The drawing under review shows one solid part. Ordinate dimensions are in mm from its lowest x, y, z. Coordinates: 2 decimals unless noted, no trailing zeros. Write each loop counter-clockwise with the first axis right and the second up, starting at its lowest first coordinate (ties: lowest second). Pieces come first, ordered by that corner, then holes. Notation, with made-up numbers: (61, 72.25) -> (79, 72.25) arc R21 cw to (79, 110.25) -> close; hole circle Ø1 at (-3, 30.5). An arc over 180 degrees is marked (long way). One line per item, written item: value. Start each with the question number.
1) Add section A-A (x = 10). State the section outline as (y, z) points.
2) Add section C-C (z = 33). State the section outline as (x, y) points.
3) For probe 1 along Z at (x, y) = (27, 0.2); probe 2 along Z at (x, y) = (37, 0.15); probe 3 along X at (y, z) = (1.9, 15.5), list the stretches that pass through material, from the lowest coordinate up. Write a range as from..to.
4) Add section B-B (y = 0.55). State the section outline as (x, z) points.
5) For pin 1 Ø0.6 at (x, y) = (12, 1) entering from -Z, flat-tipped, find the tip position at first contact; note if it passes through.
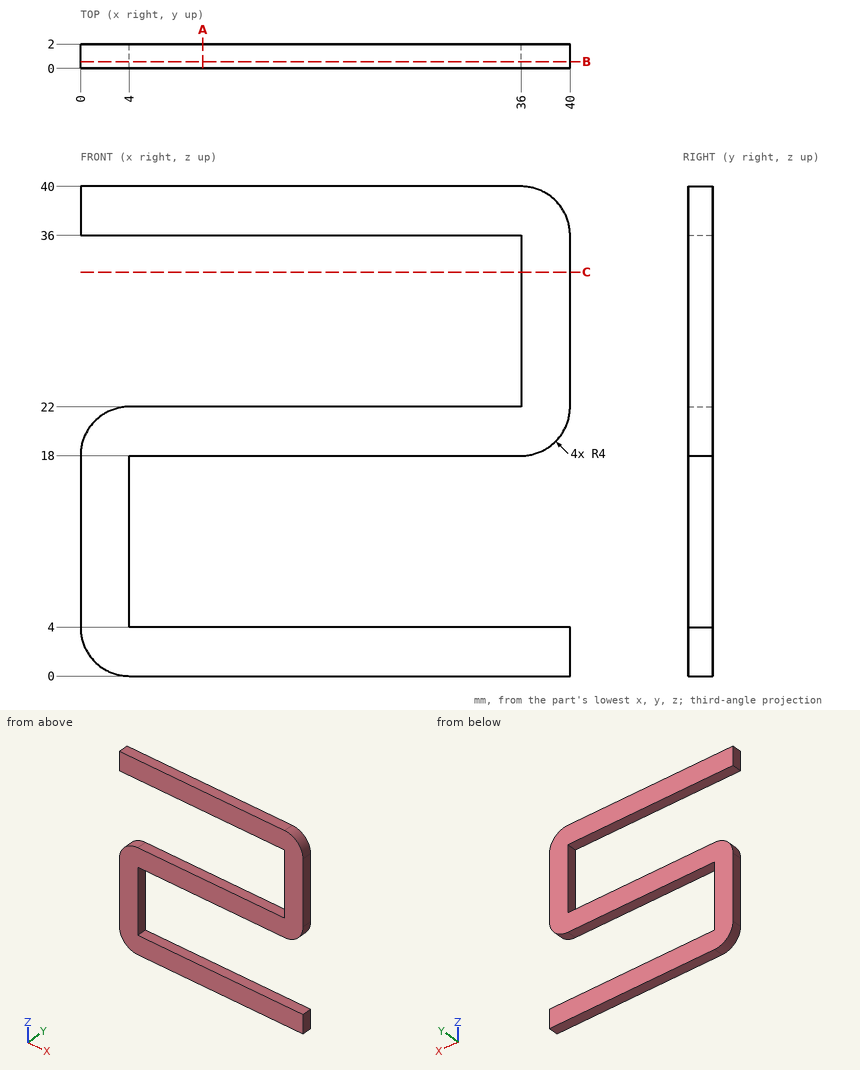
Numbers:
1. outline: (0, 0) -> (2, 0) -> (2, 4) -> (0, 4) -> close; (0, 18) -> (2, 18) -> (2, 22) -> (0, 22) -> close; (0, 36) -> (2, 36) -> (2, 40) -> (0, 40) -> close
2. outline: (36, 0) -> (40, 0) -> (40, 2) -> (36, 2) -> close
3. probe 1: 0..4, 18..22, 36..40
3. probe 2: 0..4, 18.13..39.87
3. probe 3: 0..4
4. outline: (0, 4) arc R4 ccw to (4, 0) -> (40, 0) -> (40, 4) -> (4, 4) -> (4, 18) -> (36, 18) arc R4 ccw to (40, 22) -> (40, 36) arc R4 ccw to (36, 40) -> (0, 40) -> (0, 36) -> (36, 36) -> (36, 22) -> (4, 22) arc R4 ccw to (0, 18) -> close
5. pin 1: z = 0
